```python
from build123d import *

# Parameters (mm, degrees)
KES_EKSTR_ZYON1_DEPTH            = 70.282032303
KES_EKSTR_ZYON1_DEPTH_BACK       = 70.282032303
IZIM2_W                          = 52.915026222
IZIM2_H                          = 20
IZIM4_R                          = 26.457513111
Y_KSEKLIK_EKSTR_ZYON1_DEPTH      = 5
Y_KSEKLIK_EKSTR_ZYON5_DEPTH      = 5
Y_KSEKLIK_EKSTR_ZYON5_DEPTH_BACK = 5


with BuildPart() as part:
    # izim1 → D_nd_r1 (revolve)
    with BuildSketch(Plane.XY):
        with BuildLine():
            Line((0, 38), (0, 40))
            ThreePointArc((0, 40), (40, 0), (0, -40))
            Line((0, -40), (0, -38))
            ThreePointArc((0, -38), (38, 0), (0, 38))
        make_face()
    revolve(axis=Axis((0, 48.642187878, 0), (0, -1, 0)))

    # izim2 → Kes-Ekstr_zyon1 (cut, two sides: drawn at the far end of the back side and taken through both)
    with BuildSketch(Plane.XY.offset(-KES_EKSTR_ZYON1_DEPTH_BACK)):
        with BuildLine():
            Line((0, 0), (40, 0))
            ThreePointArc((40, 0), (10.352761804, 38.637033052), (-34.641016151, 20))
            Line((-34.641016151, 20), (0, 0))
        make_face()
        with Locations((0, -40)):
            Rectangle(IZIM2_W, IZIM2_H)
    extrude(amount=KES_EKSTR_ZYON1_DEPTH + KES_EKSTR_ZYON1_DEPTH_BACK, mode=Mode.SUBTRACT)

    # izim4 → Y_kseklik-Ekstr_zyon1 (add)
    with BuildSketch(Plane.XZ.offset(30)):
        with Locations(Location((0, 0, 0), (0, 0, 270))):
            Circle(IZIM4_R)
    extrude(amount=Y_KSEKLIK_EKSTR_ZYON1_DEPTH)

    # izim13 → Y_kseklik-Ekstr_zyon5 (add, two sides: drawn at the far end of the back side and taken through both)
    with BuildSketch(Plane.XY.offset(-Y_KSEKLIK_EKSTR_ZYON5_DEPTH_BACK)):
        with BuildLine():
            Line((-17.204650534, -35), (-31.457513111, -35))
            Line((-31.457513111, -35), (-31.457513111, -23.05265427))
            ThreePointArc((-31.457513111, -23.05265427), (-25.053668597, -29.88835375), (-17.204650534, -35))
        make_face()
    extrude(amount=Y_KSEKLIK_EKSTR_ZYON5_DEPTH + Y_KSEKLIK_EKSTR_ZYON5_DEPTH_BACK)


solid = part.part
```
Could you check a few things on this model? Use its own coordinates, in mm. A direction names the side the tool comes from. Round coordinates to 2 decimals unless told otherwise and drop trailing zeros. Order: outer loops, then holes, each group sorted by start corner. A loop starts at its lowest first (then second) coordinate and runs counter-clockwise, first axis right, second up. Notation, with made-up numbers: (-22.75, 15.5) -> (2.25, 15.5) arc R19 cw to (2.25, 42.5) -> close; hole circle Ø7 at (64, 55.25). An arc over 180 degrees is marked (long way). One line per question, with ' | ' between items.
Q1. Which directions (+Z, -Z, +X, -X, +Y, -Y) give clear straight access to the entire face, cutting with the end or side of a thin tool? Please do faces 1 (the face through (-32.797, 18.936, 5.739)), 2 (the face through (26.435, -32.465, -1.093)), 3 (the face through (-29, -31, 5)).
Computed values:
face 1: +Z, -Z, +X, +Y | face 2: -Y | face 3: +Z, -X, -Y
Q2. If we section it at B-B on x = -21.5: Write out the boundary of the cut face in (y, z).
Computed values:
outline: (-35, -15.42) -> (-30, -15.42) arc R33.73 ccw to (12.41, -31.36) -> (12.41, -28.77) arc R31.33 cw to (-30, -9.04) -> (-30, 9.04) arc R31.33 cw to (12.41, 28.77) -> (12.41, 31.36) arc R33.73 ccw to (-30, 15.42) -> (-35, 15.42) -> close
Q3. I'm going to push flat-ended pins straight in: pin 1 (8 mm diameter, centred on y = -27.5, z = 2, fed in from -X); pin 2 (1.5 mm diameter, centred on x = -27, y = 9.5, fed in from -Z); pin 3 (1.5 mm diameter, centred on x = 14, y = -17.5, fed in from +Z). Where does each tip first touch, or does it pass through?
Computed values:
pin 1: x = -32.32 | pin 2: z = -28.69 | pin 3: z = 33.63
Q4. If we section it at D-D on y = 17: Write out the boundary of the cut face in (x, z), plus the area to 3 significant figures.
Computed values:
outline: (-29.44, -21.07) -> (-29.44, -16.97) arc R33.99 cw to (-29.44, 16.97) -> (-29.44, 21.07) arc R36.21 ccw to start | area: 89.7 mm²
Q5. If I drill on line 1 (X direction, y = -14.5, z = -25); line 2 (Y direction, x = 1, z = 4); line 3 (Z direction, x = -23.5, y = -25.5), over which ranges is the centre line in solid material (lowest first)? Write a range as from..to.
Computed values:
line 1: -27.65..-24.67, 24.67..27.65 | line 2: -35..-30 | line 3: -19.94..-15.54, 15.54..19.94
Q6. If we section it at A-A on z = 2: Write out the boundary of the cut face in (x, y).
Computed values:
outline: (-34.6, 19.97) arc R39.95 ccw to (-31.46, -24.63) -> (-31.46, -35) -> (26.38, -35) -> (26.38, -30) arc R39.95 ccw to (39.95, 0) -> (37.95, 0) arc R37.95 cw to (23.24, -30) -> (-23.24, -30) arc R37.95 cw to (-32.86, 18.97) -> close
Q7. If we section it at C-C on y = -27.5: Write out the boundary of the cut face in (x, z), plus the area to 3 significant figures.
Computed values:
outline: (-31.46, -5) -> (-28.61, -5) arc R29.05 ccw (long way) to (-28.61, 5) -> (-31.46, 5) -> close; hole circle Ø52.45 at (0, 0) | area: 516 mm²
Q8. We'd pull the mould along Z, two halves only. Please class faces 4 (the face through (0, -30, 0)), 5 (the face through (-29, -31, -5)), 6 (the face through (38, 0, 6)): released by +Z, released by -Z, zero draft, split by the parting line, or undercut.
Computed values:
face 4: undercut | face 5: released by -Z | face 6: zero draft
